Study the drawing (mm; zero at the part's minimum x, y, z) and answer. A direction names the side the tool comes from. Give positions to 0.01 mm unless a question says otherwise; leave off trailing zeros. Order: outer loops, then holes, each group sorted by start corner. A loop starts at its lowest first (then second) coordinate and runs counter-clockwise, first axis right, second up. Notation, with made-up numbers: (-40, 50.25) - (-23, 50.25) arc R25 ccw to (-23, 84.25) - close; hole circle Ø3 at (-26.75, -27). An arc over 180 degrees is marked (long way). Put each result on its own line as item: value.
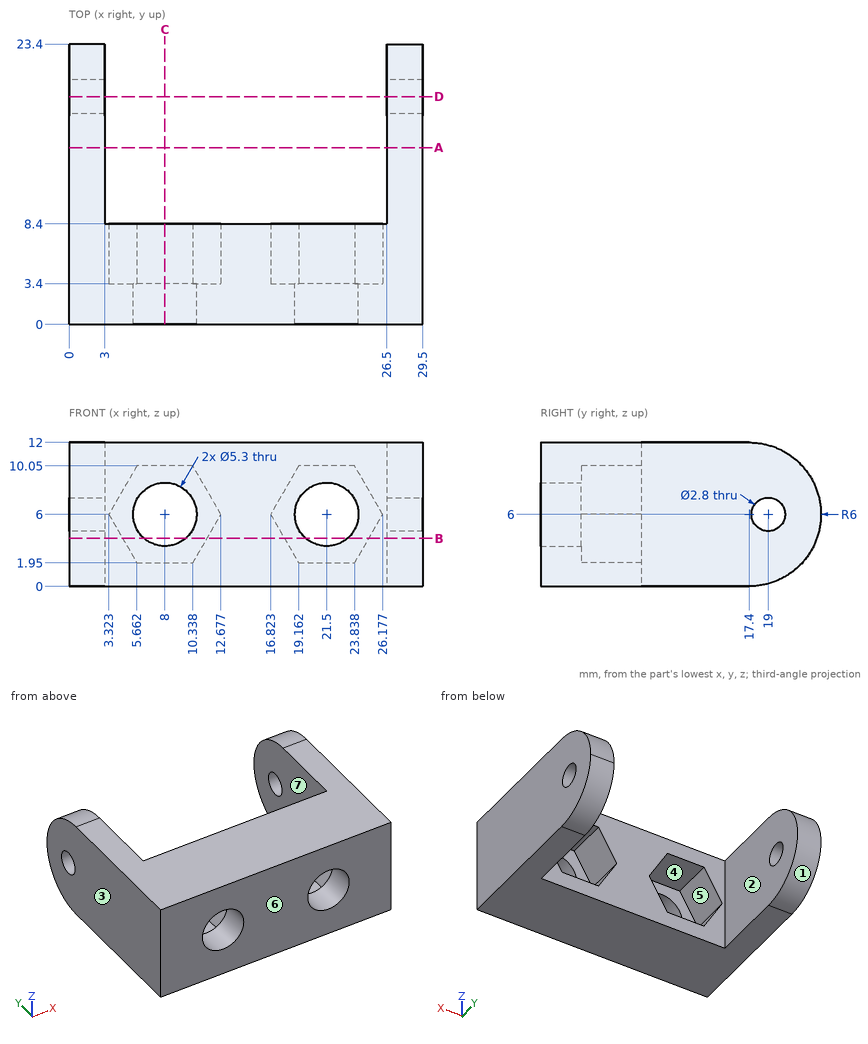
(1) A tool of negligible diameter and unlimited length cuts with its end or side. For the marked faces 5, 6 and 7, from which of +Z, -Z, +X, -X, +Y, -Y can it reach the whole face along a straight path? Write none if from no direction.
Geometry check:
face 5: +Y
face 6: +Z, -Z, +X, -X, -Y
face 7: +Z, -Z, +Y
(2) Section D-D, the plane y = 19 is taken. Write down the section's boundary in (x, z).
Geometry check:
outline: (0, 0.22) - (3, 0.22) - (3, 4.6) - (0, 4.6) - close; (0, 7.4) - (3, 7.4) - (3, 11.78) - (0, 11.78) - close; (26.5, 0.22) - (29.5, 0.22) - (29.5, 4.6) - (26.5, 4.6) - close; (26.5, 7.4) - (29.5, 7.4) - (29.5, 11.78) - (26.5, 11.78) - close
(3) Given pin 1 (7 mm diameter, centred on x = 8, z = 6, fed in from +Y); pin 2 (5 mm diameter, centred on x = 21.5, z = 1.5, fed in from +Y), each flat-ended and moving along its own axis, determine where each tip first touches the part or whether it passes through.
Geometry check:
pin 1: stops at y = 3.4
pin 2: stops at y = 8.4
(4) Determine the mould class of the marked faces 1, 2, 3 and 4 for opening direction X: pulls with the +X half, pulls with the -X half, needs draft (parallel to the pull), parting line crosses it, or undercut.
Geometry check:
face 1: needs draft
face 2: undercut
face 3: pulls with the -X half
face 4: undercut
(5) Section B-B, the plane z = 4 is taken. Write down the section's boundary in (x, y), then the cut area to 3 significant figures.
Geometry check:
outline: (0, 0) - (6.26, 0) - (6.26, 3.4) - (4.48, 3.4) - (4.48, 8.4) - (3, 8.4) - (3, 23.06) - (0, 23.06) - close; (9.74, 0) - (19.76, 0) - (19.76, 3.4) - (17.98, 3.4) - (17.98, 8.4) - (11.52, 8.4) - (11.52, 3.4) - (9.74, 3.4) - close; (23.24, 0) - (29.5, 0) - (29.5, 23.06) - (26.5, 23.06) - (26.5, 8.4) - (25.02, 8.4) - (25.02, 3.4) - (23.24, 3.4) - close
area: 242 mm²
(6) Section A-A, the plane y = 14.75 is taken. Write down the section's boundary in (x, z).
Geometry check:
outline: (0, 0) - (3, 0) - (3, 12) - (0, 12) - close; (26.5, 0) - (29.5, 0) - (29.5, 12) - (26.5, 12) - close
(7) Section C-C, the plane x = 8 is taken. Write down the section's boundary in (y, z).
Geometry check:
outline: (0, 0) - (8.4, 0) - (8.4, 1.95) - (3.4, 1.95) - (3.4, 3.35) - (0, 3.35) - close; (0, 8.65) - (3.4, 8.65) - (3.4, 10.05) - (8.4, 10.05) - (8.4, 12) - (0, 12) - close
(8) Straight lines are drawn through the part: line 1 (Z direction, x = 23, y = 5.5); line 2 (Y direction, x = 27.75, z = 6); line 3 (X direction, y = 16.75, z = 5.25). For each, find the intervals that lie inside material, in ascending order.
Geometry check:
line 1: z = 0 to 1.95, 10.05 to 12
line 2: y = 0 to 17.6, 20.4 to 23.4
line 3: x = 0 to 3, 26.5 to 29.5
